Autodesk Inventor part; units mm, degrees
ref_plane "YZ Plane" through (0, 0, 0) normal (1, 0, 0) x (0, 1, 0)
ref_plane "XZ Plane" through (0, 0, 0) normal (0, 1, 0) x (-1, 0, 0)
ref_plane "XY Plane" through (0, 0, 0) normal (0, 0, 1) x (1, 0, 0)
sketch "Sketch1" plane through (0, 0, 0) normal (0, 0, 1) x (1, 0, 0)
  circle A0 centre (0, 0) radius 44.45
  line L0 (0, 44.45) -> (44.45, 44.45)
  line L1 (44.45, 44.45) -> (44.45, -44.45)
  line L2 (44.45, -44.45) -> (0, -44.45)
  line L3 (0, -44.45) -> (0, 44.45)
  dimension "d0" = 88.9
  dimension "d1" = 44.45
  dimension "d2" = 88.9
extrude "Extrusion1" add sketch "Sketch1" along normal blind 20.955
sketch "Sketch2" plane through (0, 0, 20.955) normal (0, 0, 1) x (1, 0, 0)
  arc A0 (0, 44.45) -> (0, -44.45) centre (0, 0) ccw
  circle A1 centre (0, 0) radius 31.75
  line L0 (44.45, 44.45) -> (44.45, -44.45)
  line L1 (0, 31.75) -> (44.45, 31.75)
  line L2 (44.45, 31.75) -> (44.45, -31.75)
  line L3 (44.45, -31.75) -> (0, -31.75)
  line L4 (0, -31.75) -> (0, 31.75)
  dimension "d5" = 63.5
  dimension "d6" = 63.5
  dimension "d7" = 44.45
extrude "Extrusion2" cut sketch "Sketch2" against normal blind 10.16
sketch "Sketch3" plane through (0, 0, 10.795) normal (0, 0, 1) x (1, 0, 0)
  circle A0 centre (0, 0) radius 7.62
  dimension "d10" = 15.24
extrude "Extrusion3" cut sketch "Sketch3" against normal through all
sketch "Sketch4" plane through (0, 0, 0) normal (0, 0, -1) x (-1, 0, 0)
  circle A0 centre (0, 0) radius 15.24
  dimension "d13" = 30.48
extrude "Extrusion4" cut sketch "Sketch4" against normal blind 5.08
equation "\"d1\" = 0.5 * d0"
equation "\"d2\" = d0"
equation "\"d6\" = d5"
properties part number "Chain Guard rear arm"
Geometry: final body of the model. Coordinates: model frame, mm. A direction names the side the tool comes from. Round coordinates to 2 decimals unless told otherwise and drop trailing zeros. Write each loop counter-clockwise with the first axis right and the second up, starting at its lowest first coordinate (ties: lowest second). Pieces come first, ordered by that corner, then holes. Notation, with made-up numbers: M 29.25,46 L 33.25,46 A22 ccw 33.25,53 Z; hole C 34.25,62.25 d10. An arc over 180 degrees is marked long. Write item = value, one per line.
Item 1: Section query A-A on y = 0. Return loops of the section in (x, z) (3 decimals), then the cut area to 3 significant figures.
Findings:
outline = M -44.45,0 L -15.24,0 L -15.24,5.08 L -7.62,5.08 L -7.62,10.795 L -31.75,10.795 L -31.75,20.955 L -44.45,20.955 Z; M 7.62,5.08 L 15.24,5.08 L 15.24,0 L 44.45,0 L 44.45,10.795 L 7.62,10.795 Z
area = 847 mm^2
Item 2: Pull-direction query (Y, two-part tool) for faces 1 (the face through (22, 44.45, 10)), 2 (the face through (19, 1, 0)), 3 (the face through (23, -31.75, 16)), 4 (the face through (-44.44, -0.98, 10.33)); classes: pulls with the +Y half, pulls with the -Y half, needs draft (parallel to the pull), parting line crosses it, or undercut.
Findings:
face_1 = pulls with the +Y half
face_2 = needs draft
face_3 = undercut
face_4 = parting line crosses it
Item 3: Access query for faces 5 (the face through (44.45, 1, 8)), 6 (the face through (-31.742, 0.698, 15.946)), 7 (the face through (7, 4, 5.08)). Directions: +Z, -Z, +X, -X, +Y, -Y. A direction counts if a zero-diameter tool reaches every point of the face in a straight line with its end or side. Return the directions, or none.
Findings:
face_5 = +Z, -Z, +X, +Y, -Y
face_6 = +Z, +X
face_7 = -Z
Item 4: Material intervals for line 1 along Y through (x, z) = (0, 3.5); line 2 along Y through (x, z) = (34.5, 14.25); line 3 along Z through (x, y) = (0, 27.5) (3 decimals), sorted ascending. Write a range as [from, to].
Findings:
line_1 = [-44.45, -15.24], [15.24, 44.45]
line_2 = [-44.45, -31.75], [31.75, 44.45]
line_3 = [0, 10.795]
Item 5: Pin query (flat end, axial travel): P1, Ø10, axis at y = -21, z = 11.5, coming from the -X side; P2, Ø3, axis at x = -20, z = 12, coming from the -Y side; P3, Ø5, axis at y = -8.5, z = 17.5, coming from the -X side. Return the tip coordinate at first contact, or that it passes through.
Findings:
P1 = -41.47
P2 = -40.42
P3 = -44.04
Item 6: Section query B-B on x = 38.5. Return loops of the section in (y, z) (3 decimals), then the cut area to 3 significant figures.
Findings:
outline = M -44.45,0 L 44.45,0 L 44.45,20.955 L 31.75,20.955 L 31.75,10.795 L -31.75,10.795 L -31.75,20.955 L -44.45,20.955 Z
area = 1,220 mm^2
Item 7: Section query D-D on y = -21. Return loops of the section in (x, z) (3 decimals), then the cut area to 3 significant figures.
Findings:
outline = M -39.177,0 L 44.45,0 L 44.45,10.795 L -23.813,10.795 L -23.813,20.955 L -39.177,20.955 Z
area = 1,060 mm^2
Item 8: Section query C-C on z = 2. Return loops of the section in (x, y), then the cut area to 3 significant figures.
Findings:
outline = M 0,-44.45 L 44.45,-44.45 L 44.45,44.45 L 0,44.45 A44.45 ccw Z; hole C 0,0 d30.48
area = 6,330 mm^2
